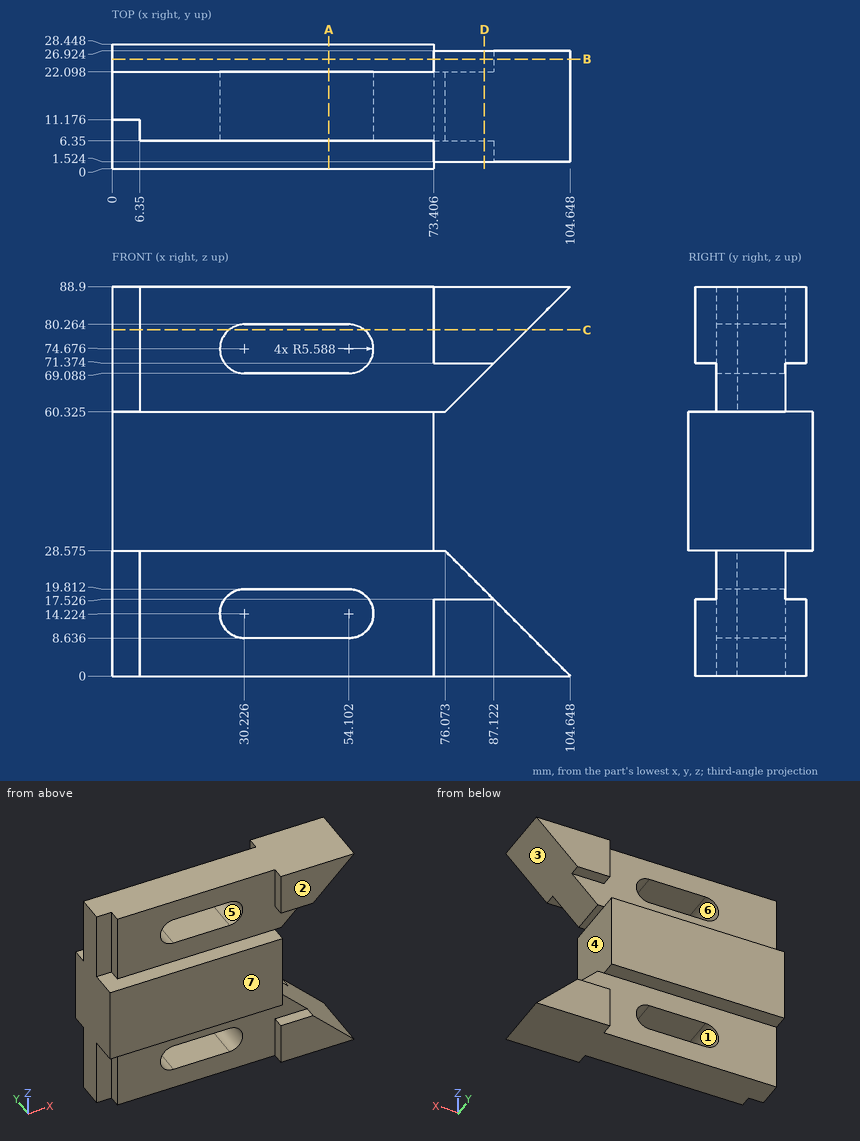
The drawing under review shows one solid part. Ordinate dimensions are in mm from its lowest x, y, z. A direction names the side the tool comes from. Round coordinates to 2 decimals unless told otherwise and drop trailing zeros. Write each loop counter-clockwise with the first axis right and the second up, starting at its lowest first coordinate (ties: lowest second). Pieces come first, ordered by that corner, then holes. Notation, with made-up numbers: (0.25, 24) -> (40.25, 24) arc R8 cw to (40.25, 36) -> close; hole circle Ø7 at (77, 76). An arc over 180 degrees is marked (long way). One line per question, with ' | ' between items. Start each with the question number.
(1) Add section A-A, the plane x = 49.5. Write out the cut boundary in (y, z) (3 decimals).
(2) Add section D-D, the plane x = 85. Write out the cut boundary in (y, z).
(3) Add section C-C, the plane z = 79. Write out the cut boundary in (x, y), plus the area to 3 significant figures.
(4) For line 1 along Z through (x, y) = (96, 20.25); line 2 along Z through (x, y) = (26.5, 18.75); line 3 along Z through (x, y) = (31, 10.5), list the stretches that pass through material, from the lowest coordinate up. Write a range as from..to.
(5) Add section B-B, the plane y = 25. Write out the cut boundary in (x, z) (3 decimals).
(6) Mouldability with a two-part tool opening along X and no side actions: class the marked faces 4, 5, 6 and 7 as released by +X, released by -X, zero draft, split by the parting line, or undercut.
(7) Insertion check: P1, Ø1.4, axis at y = 8.5, z = 73.5, coming from the -X side; P2, Ø7, axis at x = 3, z = 74, coming from the -Y side; P3, Ø10, axis at x = 58, z = 21.5, coming from the +Y side. Each pin has a flat end and moves straight along its axis. Give the tip position at first contact, or say it passes through.
(8) Tool access review of the marked faces 1, 2 and 3: name each direction out of +Z, -Z, +X, -X, +Y, -Y from which nothing blocks a thin tool from reaching the whole face with its end or side.
Answer list:
1) outline: (0, 28.575) -> (6.35, 28.575) -> (6.35, 19.812) -> (22.098, 19.812) -> (22.098, 28.575) -> (28.448, 28.575) -> (28.448, 60.325) -> (22.098, 60.325) -> (22.098, 69.088) -> (6.35, 69.088) -> (6.35, 60.325) -> (0, 60.325) -> close; (6.35, 0) -> (22.098, 0) -> (22.098, 8.636) -> (6.35, 8.636) -> close; (6.35, 80.264) -> (22.098, 80.264) -> (22.098, 88.9) -> (6.35, 88.9) -> close
2) outline: (1.52, 0) -> (26.92, 0) -> (26.92, 17.53) -> (22.1, 17.53) -> (22.1, 19.65) -> (6.35, 19.65) -> (6.35, 17.53) -> (1.52, 17.53) -> close; (1.52, 71.37) -> (6.35, 71.37) -> (6.35, 69.25) -> (22.1, 69.25) -> (22.1, 71.37) -> (26.92, 71.37) -> (26.92, 88.9) -> (1.52, 88.9) -> close
3) outline: (0, 11.18) -> (6.35, 11.18) -> (6.35, 6.35) -> (26.69, 6.35) -> (26.69, 22.1) -> (0, 22.1) -> close; (57.64, 6.35) -> (73.41, 6.35) -> (73.41, 1.52) -> (94.75, 1.52) -> (94.75, 26.92) -> (73.41, 26.92) -> (73.41, 22.1) -> (57.64, 22.1) -> close | area: 1,180 mm²
4) line 1: 0..8.65, 80.25..88.9 | line 2: 0..10.06, 18.39..70.51, 78.84..88.9 | line 3: 0..8.64, 19.81..69.09, 80.26..88.9
5) outline: (0, 28.575) -> (73.406, 28.575) -> (73.406, 60.325) -> (0, 60.325) -> close; (73.406, 0) -> (104.648, 0) -> (87.122, 17.526) -> (73.406, 17.526) -> close; (73.406, 71.374) -> (87.122, 71.374) -> (104.648, 88.9) -> (73.406, 88.9) -> close
6) face 4: released by +X | face 5: undercut | face 6: undercut | face 7: zero draft
7) P1: x = 6.35 | P2: y = 6.35 | P3: y = 22.1
8) face 1: +Y, -Y | face 2: +Z, -Z, +X, -X, -Y | face 3: +X, +Y, -Y
